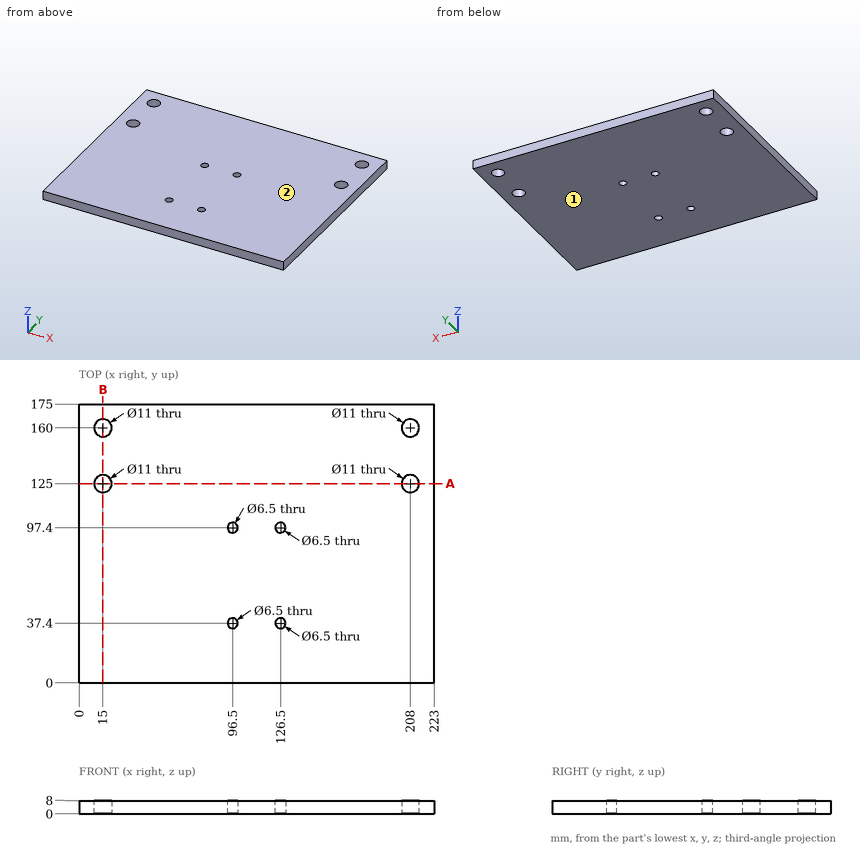
Print and shaded views of the part. All mm, measured from the part's lowest x, y and z. Round coordinates to 2 decimals unless told otherwise and drop trailing zeros. Write each loop counter-clockwise with the first axis right and the second up, starting at its lowest first coordinate (ties: lowest second). Pieces come first, ordered by that corner, then holes. Notation, with made-up numbers: (65.5, 85) -> (116.5, 85) arc R17 ccw to (116.5, 109) -> close; hole circle Ø8 at (-9.75, 29.25). An arc over 180 degrees is marked (long way). Return JSON: item names as keys, results as strings. Group by question number.
Q1. Saw through at A-A on y = 125. Write the cut outline in (x, z).
Q2. Mould opens along Z. For the marked faces 1 and 2 say: pulls with the +Z half, pulls with the -Z half, needs draft (parallel to the pull), parting line crosses it, or undercut.
Q3. Pin check, flat tips, straight feed: pin 1 (6 mm diameter, centred on x = 96.5, y = 37.4, fed in from +Z); pin 2 (17.5 mm diameter, centred on x = 15, y = 160, fed in from -Z). Stop position of each tip, or through.
Q4. Probe L1, parallel to Y at x = 208, z = 5; L2, parallel to Y at x = 127, z = 2; L3, parallel to X at y = 160, z = 4.25. List the from-to ranges inside material, lowest first. Write a range as [from, to].
Q5. Saw through at B-B on x = 15. Write the cut outline in (y, z), plus the area to 3 significant figures.
Answer:
{
 "1": {"outline": "(0, 0) -> (9.5, 0) -> (9.5, 8) -> (0, 8) -> close; (20.5, 0) -> (202.5, 0) -> (202.5, 8) -> (20.5, 8) -> close; (213.5, 0) -> (223, 0) -> (223, 8) -> (213.5, 8) -> close"},
 "2": {"face 1": "pulls with the -Z half", "face 2": "pulls with the +Z half"},
 "3": {"pin 1": "through", "pin 2": "z = 0"},
 "4": {"L1": "[0, 119.5], [130.5, 154.5], [165.5, 175]", "L2": "[0, 34.19], [40.61, 94.19], [100.61, 175]", "L3": "[0, 9.5], [20.5, 202.5], [213.5, 223]"},
 "5": {"outline": "(0, 0) -> (119.5, 0) -> (119.5, 8) -> (0, 8) -> close; (130.5, 0) -> (154.5, 0) -> (154.5, 8) -> (130.5, 8) -> close; (165.5, 0) -> (175, 0) -> (175, 8) -> (165.5, 8) -> close", "area": "1,220 mm2"}
}
